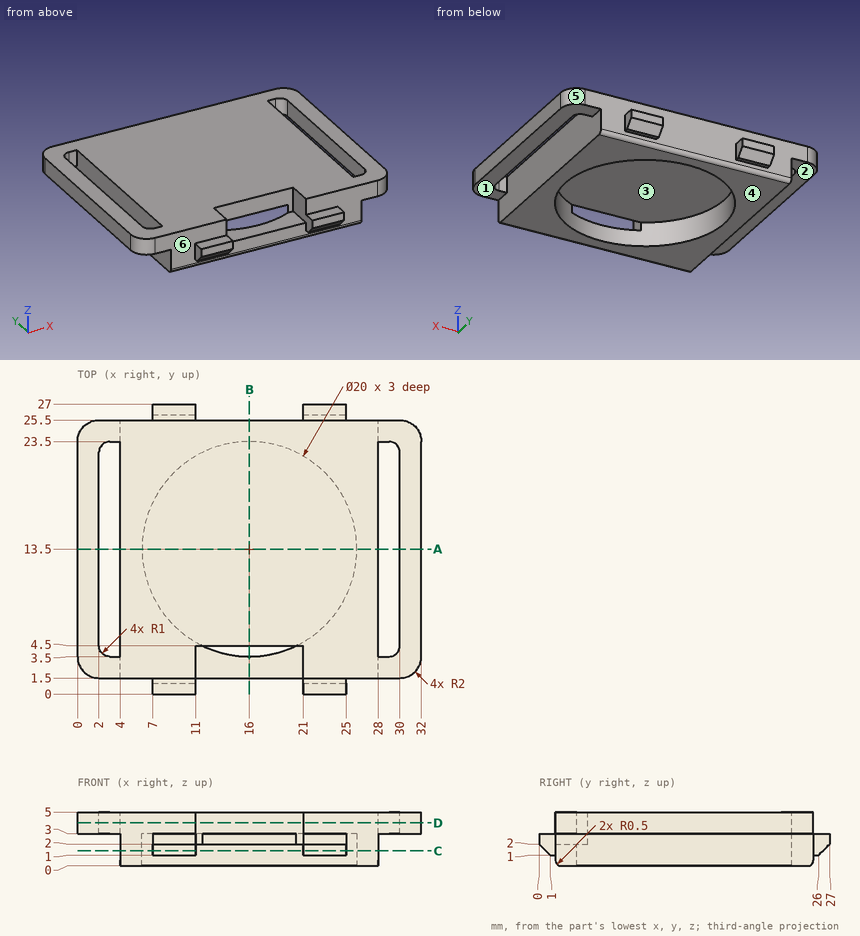
Answer from the drawing. Dimensions are ordinates in mm from the lowest x, y and z of the part. A direction names the side the tool comes from. Coordinates: 2 decimals unless noted, no trailing zeros. Loops run counter-clockwise (first coordinate to the right, second up) from the corner with the lowest first, then second, coordinate; pieces in that order, holes last. Notation, with made-up numbers: (46, -18.5) - (62, -18.5) arc R11 ccw to (62, -10.5) - close; hole circle Ø6 at (78, 82). An arc over 180 degrees is marked (long way). Use a Markdown table: item, result.
Item 1: For the marked faces 1, 2 and 3, determine the directions among +Z, -Z, +X, -X, +Y, -Y from which every point of the face is accessible in a straight line to the end or side of a thin tool.
Evaluation:
| item | result |
|---|---|
| face 1 | -Z, +X, +Y, -Y |
| face 2 | -Z, -X, +Y, -Y |
| face 3 | -Z |
Item 2: Find section A-A, the plane y = 13.5. Determine the outline of the cut face in (x, z).
Evaluation:
| item | result |
|---|---|
| outline | (0, 3) - (2, 3) - (2, 5) - (0, 5) - close; (4, 0) - (6, 0) - (6, 3) - (26, 3) - (26, 0) - (28, 0) - (28, 5) - (4, 5) - close; (30, 3) - (32, 3) - (32, 5) - (30, 5) - close |
Item 3: Given pin 1 Ø2 at (y, z) = (1, 3.5) entering from -X; pin 2 Ø0.5 at (x, z) = (3.5, 4.5) entering from +Y; pin 3 Ø2 at (y, z) = (22.5, 4) entering from -X; pin 4 Ø0.5 at (x, z) = (28.5, 4) entering from -Y, each flat-ended and moving along its own axis, determine where each tip first touches the part or whether it passes through.
Evaluation:
| item | result |
|---|---|
| pin 1 | stops at x = 0.68 |
| pin 2 | stops at y = 25.5 |
| pin 3 | stops at x = 0 |
| pin 4 | stops at y = 1.5 |
Item 4: Consider probe 1 along X at (y, z) = (16, 3.65); probe 2 along X at (y, z) = (13.5, 1.4); probe 3 along Y at (x, z) = (16, 1.1). Determine where each line is inside the solid, lowest interval first. Write a range as from..to.
Evaluation:
| item | result |
|---|---|
| probe 1 | x = 0..2, 4..28, 30..32 |
| probe 2 | x = 4..6, 26..28 |
| probe 3 | y = 1.5..3.5, 23.5..25.5 |
Item 5: Find section D-D, the plane z = 4. Determine the outline of the cut face in (x, y), and give its area (3 significant figures).
Evaluation:
| item | result |
|---|---|
| outline | (0, 3.5) arc R2 ccw to (2, 1.5) - (11, 1.5) - (11, 4.5) - (21, 4.5) - (21, 1.5) - (30, 1.5) arc R2 ccw to (32, 3.5) - (32, 23.5) arc R2 ccw to (30, 25.5) - (2, 25.5) arc R2 ccw to (0, 23.5) - close; hole (2, 4.5) arc R1 ccw to (3, 3.5) - (4, 3.5) - (4, 23.5) - (3, 23.5) arc R1 ccw to (2, 22.5) - close; hole (28, 3.5) - (29, 3.5) arc R1 ccw to (30, 4.5) - (30, 22.5) arc R1 ccw to (29, 23.5) - (28, 23.5) - close |
| area | 655 mm2 |
Item 6: Find section C-C, the plane z = 1.4. Determine the outline of the cut face in (x, y), and give its area (3 significant figures).
Evaluation:
| item | result |
|---|---|
| outline | (4, 1.5) - (7, 1.5) - (7, 0.6) - (11, 0.6) - (11, 1.5) - (21, 1.5) - (21, 0.6) - (25, 0.6) - (25, 1.5) - (28, 1.5) - (28, 25.5) - (25, 25.5) - (25, 26.4) - (21, 26.4) - (21, 25.5) - (11, 25.5) - (11, 26.4) - (7, 26.4) - (7, 25.5) - (4, 25.5) - close; hole circle Ø20 at (16, 13.5) |
| area | 276 mm2 |
Item 7: Find section B-B, the plane x = 16. Determine the outline of the cut face in (y, z).
Evaluation:
| item | result |
|---|---|
| outline | (1.5, 0.5) arc R0.5 ccw to (2, 0) - (3.5, 0) - (3.5, 2) - (1.5, 2) - close; (4.5, 3) - (23.5, 3) - (23.5, 0) - (25, 0) arc R0.5 ccw to (25.5, 0.5) - (25.5, 5) - (4.5, 5) - close |
Item 8: The mould has two halves that part along X. Classify the marked faces 4, 5 and 6: +X half, -X half, draft (parallel to the pull), parting line (faces both ways), or undercut.
Evaluation:
| item | result |
|---|---|
| face 4 | draft |
| face 5 | +X half |
| face 6 | undercut |
